from build123d import *

# Parameters (mm, degrees)
EXTRUDE_START         = -12.47
EXTRUDE_1_DEPTH       = 23.94
EXTRUDE_START_2       = -42.420417041
EXTRUDE_3_DEPTH       = 42.420417041
EXTRUDE_START_3       = 135
EXTRUDE_3_2_OUTLINE_W = 5.53
EXTRUDE_3_2_OUTLINE_H = 12
EXTRUDE_3_2_DEPTH     = 1
EXTRUDE_START_4       = 92.811966442
EXTRUDE_3_3_OUTLINE_W = 5.53
EXTRUDE_3_3_OUTLINE_H = 12
EXTRUDE_3_3_DEPTH     = 0.418113953
SKETCH_3_W            = 8.92360814
SKETCH_3_H            = 8.098758973
CUT_EXTRUDE_1_DEPTH   = 24.94
EXTRUDE_4_DEPTH       = 4
EXTRUDE_5_DEPTH       = 1
FILLET_1_R            = 3
CUT_EXTRUDE_START     = -12.47
CUT_EXTRUDE_4_DEPTH   = 20.17
CUT_EXTRUDE_START_2   = 130.027390523
CUT_EXTRUDE_4_2_DEPTH = 4.972609477
CUT_EXTRUDE_5_REACH   = 78.971
SKETCH_6_R            = 1.6
CUT_EXTRUDE_6_DEPTH   = 8.2
CUT_EXTRUDE_8_DEPTH   = 10


with BuildPart() as part:
    # 草图1 → 凸台-拉伸1 (new body)
    with BuildSketch(Plane(origin=(0, 0, 0), x_dir=(0, 0, -1), z_dir=(1, 0, 0)).offset(EXTRUDE_START)):
        Polygon((-135, 224), (-135, 206.75), (-116.178095192, 206.75), (-104.005, 198.85), (-104.005, 168.99910251), (-93.25, 163.930391323), (-93.25, 219.611898178), align=None)
    extrude(amount=EXTRUDE_1_DEPTH)

    # 凸台-拉伸3: read off the stored shape, not the designer's step
    # 凸台-拉伸3 outline → 凸台-拉伸3 (add)
    with BuildSketch(Plane(origin=(11.47, 224, 135), x_dir=(1, 0, 0), z_dir=(0, 0.10452846326765014, 0.9945218953682736)).offset(EXTRUDE_START_2)):
        with BuildLine():
            Line((0, 0), (0, -4))
            Line((0, -4), (4, -4))
            ThreePointArc((4, -4), (2.828427125, -1.171572875), (0, 0))
        make_face()
    extrude(amount=EXTRUDE_3_DEPTH)

    # Extrude 3 2 outline → Extrude 3 2 (cut)
    with BuildSketch(Plane.XY.offset(EXTRUDE_START_3)):
        with Locations((14.235, 220)):
            Rectangle(EXTRUDE_3_2_OUTLINE_W, EXTRUDE_3_2_OUTLINE_H)
    extrude(amount=EXTRUDE_3_2_DEPTH, mode=Mode.SUBTRACT)

    # Extrude 3 3 outline → Extrude 3 3 (cut)
    with BuildSketch(Plane.XY.offset(EXTRUDE_START_4)):
        with Locations((14.235, 220)):
            Rectangle(EXTRUDE_3_3_OUTLINE_W, EXTRUDE_3_3_OUTLINE_H)
    extrude(amount=EXTRUDE_3_3_DEPTH, mode=Mode.SUBTRACT)

    # 草图3 → 切除-拉伸1 (cut)
    with BuildSketch(Plane(origin=(0, 0, 93.25), x_dir=(-1, 0, 0), z_dir=(0, 0, -1))):
        with Locations((-14.443820209, 216.390986059)):
            Rectangle(SKETCH_3_W, SKETCH_3_H)
    extrude(amount=CUT_EXTRUDE_1_DEPTH, mode=Mode.SUBTRACT)

    # 草图4 → 凸台-拉伸4 (add)
    with BuildSketch(Plane(origin=(11.47, 0, 0), x_dir=(0, 0, -1), z_dir=(1, 0, 0))):
        Polygon((-93.25, 206.75), (-93.25, 215.589865059), (-135, 219.977966882), (-135, 206.75), align=None)
    extrude(amount=EXTRUDE_4_DEPTH)

    # 草图10 → 凸台-拉伸5 (add)
    with BuildSketch(Plane(origin=(11.47, 0, 0), x_dir=(0, 0, -1), z_dir=(1, 0, 0))):
        Polygon((-93.25, 163.930391323), (-104.005, 168.99910251), (-104.005, 198.85), (-116.178095192, 206.75), (-93.25, 206.75), align=None)
    extrude(amount=EXTRUDE_5_DEPTH)

    # 圆角1
    fillet_1_edges = [part.edges().sort_by_distance(p)[0] for p in [
        (-12.47, 215.375, 135),
    ]]
    fillet(fillet_1_edges, radius=FILLET_1_R)

    # 切除-拉伸4: read off the stored shape, not the designer's step
    # 切除-拉伸4 outline → 切除-拉伸4 (cut)
    with BuildSketch(Plane.YZ.offset(CUT_EXTRUDE_START)):
        Polygon((210.75, 131.365089719), (223.477357684, 130.027390523), (224, 135), (210.75, 135), align=None)
    extrude(amount=CUT_EXTRUDE_4_DEPTH, mode=Mode.SUBTRACT)

    # Cut-Extrude 4 2 outline → Cut-Extrude 4 2 (add)
    with BuildSketch(Plane.XY.offset(CUT_EXTRUDE_START_2)):
        with BuildLine():
            ThreePointArc((7.7, 213.75), (6.821320344, 211.628679656), (4.7, 210.75))
            Line((4.7, 210.75), (7.7, 210.75))
            Line((7.7, 210.75), (7.7, 213.75))
        make_face()
    extrude(amount=CUT_EXTRUDE_4_2_DEPTH)

    # 切除-拉伸5: up to this plane
    cut_extrude_5_end = Plane(origin=(11.47, 219.611898178, 93.25), z_dir=(0, 0, 1))
    # 草图6 → 切除-拉伸5 (cut, up to the surface)
    with BuildSketch(Plane(origin=(11.47, 224, 135), x_dir=(1, 0, 0), z_dir=(0, 0.10452846326765014, 0.9945218953682736)), mode=Mode.PRIVATE) as cut_extrude_5_sk1:
        with Locations(Location((0, -4, 0), (0, 0, 90))):
            Circle(SKETCH_6_R)
    cut_extrude_5_tool1 = split(extrude(cut_extrude_5_sk1.sketch, amount=-CUT_EXTRUDE_5_REACH, mode=Mode.PRIVATE), bisect_by=cut_extrude_5_end, keep=Keep.BOTH, mode=Mode.PRIVATE)
    add(cut_extrude_5_tool1.solids().sort_by_distance((11.47, 220.021912, 135.418114))[0], mode=Mode.SUBTRACT)

    # 草图7 → 切除-拉伸6 (cut)
    with BuildSketch(Plane(origin=(0, 207.518492152, -21.811072421), x_dir=(1, 0, 0), z_dir=(0, 0.9945218953682738, -0.10452846326765014))):
        with BuildLine():
            Line((15.47, -149.674831647), (15.47, -122.694860975))
            Line((15.47, -122.694860975), (-4.7, -122.694860975))
            ThreePointArc((-4.7, -122.694860975), (-6.821320344, -123.573540631), (-7.7, -125.694860975))
            Line((-7.7, -125.694860975), (-7.7, -146.674831647))
            ThreePointArc((-7.7, -146.674831647), (-6.821320344, -148.79615199), (-4.7, -149.674831647))
            Line((-4.7, -149.674831647), (15.47, -149.674831647))
        make_face()
    extrude(amount=-CUT_EXTRUDE_6_DEPTH, mode=Mode.SUBTRACT)

    # 草图9 → 切除-拉伸8 (cut)
    with BuildSketch(Plane.ZY.offset(12.47)):
        with BuildLine():
            Line((122.934325929, 219.212567575), (114.978150766, 218.376339869))
            ThreePointArc((114.978150766, 218.376339869), (113.969224519, 217.828537613), (113.643160618, 216.727764331))
            Line((113.643160618, 216.727764331), (113.768594774, 215.534338057))
            ThreePointArc((113.768594774, 215.534338057), (114.316397031, 214.52541181), (115.417170312, 214.199347909))
            Line((115.417170312, 214.199347909), (123.373345475, 215.035575615))
            ThreePointArc((123.373345475, 215.035575615), (124.382271722, 215.583377871), (124.708335623, 216.684151153))
            Line((124.708335623, 216.684151153), (124.582901467, 217.877577427))
            ThreePointArc((124.582901467, 217.877577427), (124.035099211, 218.886503674), (122.934325929, 219.212567575))
        make_face()
    extrude(amount=-CUT_EXTRUDE_8_DEPTH, mode=Mode.SUBTRACT)


solid = part.part
Can you work these out from the model? Positions are in its coordinate system, mm. A direction names the side the tool comes from. Coordinates: 2 decimals unless noted, no trailing zeros. Loops run counter-clockwise (first coordinate to the right, second up) from the corner with the lowest first, then second, coordinate; pieces in that order, holes last. Notation, with made-up numbers: (52.5, 38) - (69.5, 38) arc R26 ccw to (69.5, 55) - close; hole circle Ø7 at (50, 3). An arc over 180 degrees is marked (long way). Answer as a JSON object with one key per item and string values. Group by question number.
Item 1: If we section it at B-B (x = 1): List the corners of the cut face in (y, z) for me (3 decimals).
Item 2: If we mould it in two halves opening along Z, with no side actions, what happens to faces 1 (the face through (-10.1, 218.8, 119)), 2 (the face through (1, 206.75, 124)), 3 (the face through (14.329, 218.754, 96.596))? For each: released by +Z, released by -Z, zero draft, split by the parting line, or undercut.
Item 3: For pin 1 (7 mm diameter, centred on y = 190.5, z = 100, fed in from +X); pin 2 (5 mm diameter, centred on y = 217, z = 114.5, fed in from +X); pin 3 (10 mm diameter, centred on x = -9, y = 172, fed in from +Z) (3 decimals), each with a flat end and sliding along its axis, tell me the tip position at first contact or that it passes through.
Item 4: If we section it at C-C (z = 105.5): List the corners of the cut face in (x, y) for me, plus the area to 3 significant figures.
Item 5: If I drill on L1, parallel to X at y = 201, z = 98; L2, parallel to Z at x = 8.5, y = 183 (3 decimals); L3, parallel to Y at x = -7, z = 127, over which ranges is the centre line in solid material (lowest first)? Write a range as from..to.
Item 6: On a 3-axis mill with a long thin cutter (end or side, diameter ignored), from which of +Z, -Z, +X, -X, +Y, -Y can I reach the whole of each face in a straight line? I mean faces 4 (the face through (-6.8, 216.41, 101.49)), 5 (the face through (12.47, 190, 99)), 6 (the face through (-10.118, 217.273, 124.646)). Say none if no direction works.
Item 7: If we section it at A-A (z = 121.5): List the corners of the cut face in (x, y) for me, plus the area to 3 significant figures.
Item 8: If we section it at D-D (y = 189): List the corners of the cut face in (x, z) for me (3 decimals).
Returned:
{
 "1": {"outline": "(163.93, 93.25) - (219.612, 93.25) - (220.344, 100.212) - (212.189, 101.069) - (215.009, 127.901) - (223.164, 127.044) - (223.477, 130.027) - (210.75, 131.365) - (210.75, 135) - (206.75, 135) - (206.75, 116.178) - (198.85, 104.005) - (168.999, 104.005) - close"},
 "2": {"face 1": "undercut", "face 2": "zero draft", "face 3": "released by -Z"},
 "3": {"pin 1": "stops at x = 12.47", "pin 2": "stops at x = -7.7", "pin 3": "stops at z = 104.005"},
 "4": {"outline": "(-12.47, 199.82) - (12.47, 199.82) - (12.47, 206.75) - (15.47, 206.75) - (15.47, 212.65) - (-7.7, 212.65) - (-7.7, 220.9) - (-12.47, 220.9) - close", "area": "377 mm²"},
 "5": {"L1": "x = -12.47..12.47", "L2": "z = 93.25..104.005", "L3": "y = 206.75..223.16"},
 "6": {"face 4": "+X, +Y", "face 5": "+Z, -Z, +X, -Y", "face 6": "+X, -X"},
 "7": {"outline": "(-12.47, 206.75) - (15.47, 206.75) - (15.47, 214.34) - (-7.7, 214.34) - (-7.7, 214.84) - (-12.47, 214.84) - close; (-12.47, 219.06) - (-7.7, 219.06) - (-7.7, 222.58) - (-12.47, 222.58) - close", "area": "231 mm²"},
 "8": {"outline": "(-12.47, 93.25) - (12.47, 93.25) - (12.47, 104.005) - (-12.47, 104.005) - close"}
}
